Source: CAD feature listing. Evaluate the final solid. Frame: model axes, mm. Face numbers are marked on the shaded views. A direction names the side the tool comes from. Give positions to 0.01 mm unless a question says otherwise; leave off trailing zeros. Write each loop counter-clockwise with the first axis right and the second up, starting at its lowest first coordinate (ties: lowest second). Pieces come first, ordered by that corner, then holes. Notation, with made-up numbers: (62.5, 54) -> (96.5, 54) arc R26 ccw to (96.5, 68) -> close; hole circle Ø7 at (89, 23.25). An arc over 180 degrees is marked (long way). Write item = value, one per line.
from build123d import *

# Parameters (mm, degrees)
BOSS_EXTRUDE1_DEPTH = 2


with BuildPart() as part:
    # Sketch1 → Boss-Extrude1 (new body)
    with BuildSketch(Plane(origin=(0, 0, 0), x_dir=(1, 0, 0), z_dir=(0, 1, 0))):
        with BuildLine():
            ThreePointArc((0, 3.5), (-1.984314586, 2.88313989), (-3.269175164, 1.2499975))
            Line((-3.269175164, 1.2499975), (-0.630480967, 1.2499975))
            ThreePointArc((-0.630480967, 1.2499975), (1.4, 0), (-0.630480967, -1.2499975))
            Line((-0.630480967, -1.2499975), (-3.269175164, -1.2499975))
            ThreePointArc((-3.269175164, -1.2499975), (-1.984314586, -2.88313989), (0, -3.5))
            Line((0, -3.5), (10.16, -3.5))
            ThreePointArc((10.16, -3.5), (11.956051224, -2.756051224), (12.7, -0.96))
            Line((12.7, -0.96), (12.7, 0.96))
            ThreePointArc((12.7, 0.96), (11.956051224, 2.756051224), (10.16, 3.5))
            Line((10.16, 3.5), (0, 3.5))
        make_face()
    extrude(amount=BOSS_EXTRUDE1_DEPTH)


solid = part.part
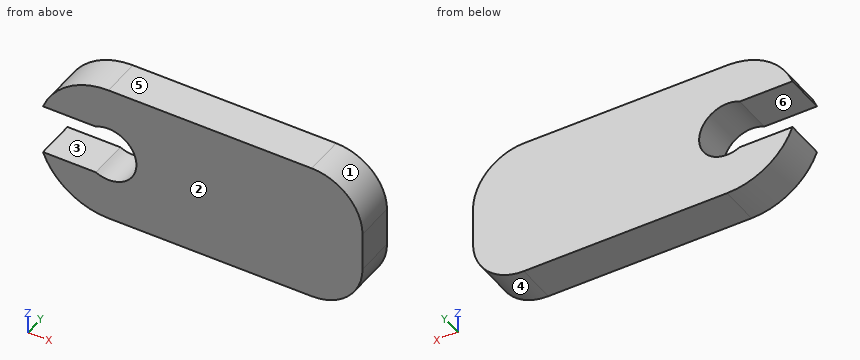
(1) Access query for the marked faces 5 and 6. Directions: +Z, -Z, +X, -X, +Y, -Y. A direction counts if a zero-diameter tool reaches every point of the face in a straight line with its end or side. Return the directions, or none.
Values follow:
face_5 = +Z, +X, -X, +Y, -Y
face_6 = -X, +Y, -Y
(2) Section query B-B (z = 0). Return loops of the section in (x, y).
Values follow:
outline = (1.4, 0) -> (12.7, 0) -> (12.7, 2) -> (1.4, 2) -> close
(3) First-contact query: pin 1 (1.7 mm diameter, centred on x = 0, z = 0, fed in from +Y); pin 2 (1 mm diameter, centred on x = -1.5, y = 1, fed in from +Z). Flat tips, straight axial feed; report the tip coordinate or a pass-through.
Values follow:
pin_1 = through
pin_2 = 3.35
(4) Material intervals for line 1 (Z direction, x = 0, y = 1.25); line 2 (X direction, y = 1.5, z = 0); line 3 (Z direction, x = 0.75, y = 1.25), sorted ascending.
Values follow:
line_1 = -3.5 to -1.4, 1.4 to 3.5
line_2 = 1.4 to 12.7
line_3 = -3.5 to -1.18, 1.18 to 3.5
(5) Section query A-A (y = 1.1). Return loops of the section in (x, z), plus the area to 3 significant figures.
Values follow:
outline = (-3.27, -1.25) arc R3.5 ccw to (0, -3.5) -> (10.16, -3.5) arc R2.54 ccw to (12.7, -0.96) -> (12.7, 0.96) arc R2.54 ccw to (10.16, 3.5) -> (0, 3.5) arc R3.5 ccw to (-3.27, 1.25) -> (-0.63, 1.25) arc R1.4 cw (long way) to (-0.63, -1.25) -> close
area = 93.6 mm2
(6) Section query C-C (z = 0.75). Return loops of the section in (x, y).
Values follow:
outline = (1.18, 0) -> (12.7, 0) -> (12.7, 2) -> (1.18, 2) -> close
(7) Pull-direction query (Z, two-part tool) for the marked faces 1, 2, 3 and 4; classes: pulls with the +Z half, pulls with the -Z half, needs draft (parallel to the pull), parting line crosses it, or undercut.
Values follow:
face_1 = pulls with the +Z half
face_2 = needs draft
face_3 = undercut
face_4 = pulls with the -Z half
